Check sheet for the modelled part. Datum: model origin and axes. Units: mm. A direction names the side the tool comes from. Round coordinates to 2 decimals unless told otherwise and drop trailing zeros. Loops run counter-clockwise (first coordinate to the right, second up) from the corner with the lowest first, then second, coordinate; pieces in that order, holes last. Notation, with made-up numbers: (-34.75, -3.75) -> (16.25, -3.75) arc R12 ccw to (16.25, 14.25) -> close; hole circle Ø9 at (-8.5, -22). An arc over 180 degrees is marked (long way). Return JSON: item names as keys, results as strings.
from build123d import *

# Parameters (mm, degrees)
F0_W     = 242.720081
F0_H     = 300.530582
F1_DEPTH = 25.4


with BuildPart() as f1:
    # F0 (on Front) → F1 (new body)
    with BuildSketch(Plane.XZ):
        Polygon((-120.807813, 291.692996), (-438.307813, 291.692996), (-438.307813, -165.507004), (-120.807813, -165.507004), (158.94197, 35.91284), (196.692187, 63.092996), (160.690517, 89.014198), align=None)
        with Locations((-242.167854, 64.014867)):
            Rectangle(F0_W, F0_H, mode=Mode.SUBTRACT)
        with BuildLine():
            ThreePointArc((196.692187, 91.555874), (178.323721, 95.492349), (160.690517, 89.014198))
            Line((160.690517, 89.014198), (196.692187, 63.092996))
            Line((196.692187, 63.092996), (196.692187, 91.555874))
        make_face()
        with BuildLine():
            Line((196.692187, 91.555874), (196.692187, 63.092996))
            Line((196.692187, 63.092996), (196.692187, 31.995555))
            ThreePointArc((196.692187, 31.995555), (214.504632, 61.775715), (196.692187, 91.555874))
        make_face()
        with BuildLine():
            Line((196.692187, 31.995555), (196.692187, 63.092996))
            Line((196.692187, 63.092996), (158.94197, 35.91284))
            ThreePointArc((158.94197, 35.91284), (177.215375, 28.155683), (196.692187, 31.995555))
        make_face()
    extrude(amount=F1_DEPTH)


solid = f1.part
Q1. Section check B-B (y = -11.25). Record the boundary of the cut face in (x, z).
Results list:
{"outline": "(-438.31, -165.51) -> (-120.81, -165.51) -> (158.94, 35.91) arc R33.8 ccw to (196.69, 32) arc R33.8 ccw to (196.69, 91.56) arc R33.8 ccw to (160.69, 89.01) -> (-120.81, 291.69) -> (-438.31, 291.69) -> close; hole (-363.53, -86.25) -> (-120.81, -86.25) -> (-120.81, 214.28) -> (-363.53, 214.28) -> close"}
Q2. Tool access check on faces 1 (the flat face through (-116, -25.4, 66)), 2 (the flat face through (-244, -13, -86.25)). Record the directions out of +Z, -Z, +X, -X, +Y, -Y that give a thin tool (end or side, any length) a straight path to the whole face; none if there is none.
Results list:
{"face 1": "+Z, -Z, +X, -X, -Y", "face 2": "+Y, -Y"}
Q3. Section check C-C (z = -14). Record the boundary of the cut face in (x, y), then the cut area to 3 significant figures.
Results list:
{"outline": "(-438.31, -25.4) -> (-363.53, -25.4) -> (-363.53, 0) -> (-438.31, 0) -> close; (-120.81, -25.4) -> (89.62, -25.4) -> (89.62, 0) -> (-120.81, 0) -> close", "area": "7,240 mm^2"}
Q4. Section check D-D (x = 94). Record the boundary of the cut face in (y, z), then the cut area to 3 significant figures.
Results list:
{"outline": "(-25.4, -10.85) -> (0, -10.85) -> (0, 137.03) -> (-25.4, 137.03) -> close", "area": "3,760 mm^2"}
Q5. Section check A-A (x = -225). Record the boundary of the cut face in (y, z).
Results list:
{"outline": "(-25.4, -165.51) -> (0, -165.51) -> (0, -86.25) -> (-25.4, -86.25) -> close; (-25.4, 214.28) -> (0, 214.28) -> (0, 291.69) -> (-25.4, 291.69) -> close"}
Q6. Material ranges on line 1 (Z direction, x = -279.5, y = -18.5); line 2 (X direction, y = -14.25, z = 3); line 3 (X direction, y = -2.75, z = 84.5), recorded low to high.
Results list:
{"line 1": "-165.51 to -86.25, 214.28 to 291.69", "line 2": "-438.31 to -363.53, -120.81 to 113.23", "line 3": "-438.31 to -363.53, -120.81 to 205.73"}
Q7. Go/stop test with a flat-tipped pin: pin 1 (3 mm diameter, centred on x = -68.5, y = -6.5, fed in from -Z). Record where the tip stops, or that it passes through.
Results list:
{"pin 1": "z = -128.93"}
Q8. Draft check along Z on faces 3 (the flat face through (-120.808, -13, 62)), 4 (the flat face through (-438.308, -13, 66)), 5 (the flat face through (-277, -13, 291.693)), 6 (the flat face through (17.109, -12.522, -66.207)). Enter one of: released by +Z, released by -Z, zero draft, split by the parting line, or undercut.
Results list:
{"face 3": "undercut", "face 4": "zero draft", "face 5": "released by +Z", "face 6": "released by -Z"}
